Read the model definition and answer for the solid it produces. Units are mm, in the model's axes. Coordinates: 2 decimals unless noted, no trailing zeros. Write each loop counter-clockwise with the first axis right and the second up, starting at its lowest first coordinate (ties: lowest second). Pieces come first, ordered by that corner, then holes.
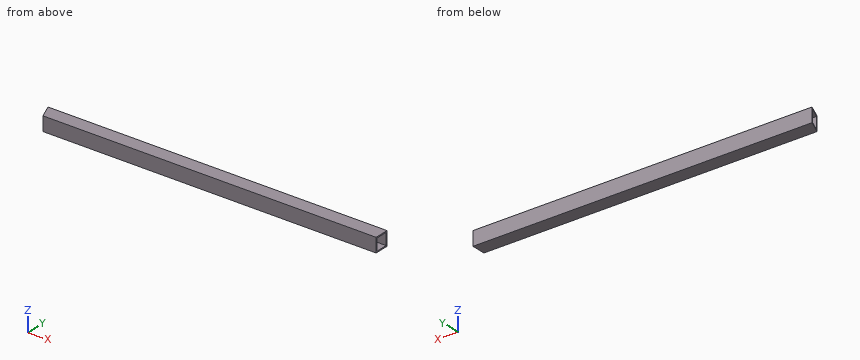
from build123d import *

# Parameters (mm, degrees)
F0_W        = 25
F0_H        = 25
F0_W_2      = 21
F0_H_2      = 21
F1_DEPTH    = 600
F2_T1_DEPTH = 180.5602235744


# Not quite as in the source:
# - a fillet or chamfer that OpenCascade refuses, or shapes differently, is made with other operations: its cross-section is extruded or revolved along the edge and cut away or added


with BuildPart() as f1:
    # F0 (on Right) → F1 (new body)
    with BuildSketch(Plane.YZ):
        Rectangle(F0_W, F0_H)
        Rectangle(F0_W_2, F0_H_2, mode=Mode.SUBTRACT)
    extrude(amount=F1_DEPTH)

    # F2: chamfer of 30 x 12.4264068712 on 1 edges, made by hand

    # F2_s2 → F2_t1 (cut)
    with BuildSketch(Plane.XY.offset(-90.2801117872)):
        Polygon((12.4264068712, -12.5), (0, 17.5), (0, -12.5), align=None)
    extrude(amount=F2_T1_DEPTH, mode=Mode.SUBTRACT)


solid = f1.part
Item 1: The part is cut by section C-C (y = -3). Give the vertices of the cut face in (x, z), and give its area (3 significant figures).
Item 2: Find the intervals of material crossed by probe 1 along Z at (x, y) = (469, 8.5); probe 2 along X at (y, z) = (-7, 10.75), in increasing order.
Item 3: The part is cut by section A-A (z = -3.75). Give the vertices of the cut face in (x, y), and give its area (3 significant figures).
Item 4: The part is cut by section B-B (x = 404.5). Give the vertices of the cut face in (y, z), and give its area (3 significant figures).
Answer:
1. outline: (8.49, -12.5) - (600, -12.5) - (600, -10.5) - (8.49, -10.5) - close; (8.49, 10.5) - (600, 10.5) - (600, 12.5) - (8.49, 12.5) - close
1. area: 2,370 mm2
2. probe 1: z = -12.5 to -10.5, 10.5 to 12.5
2. probe 2: x = 10.15 to 600
3. outline: (2.07, 12.5) - (2.9, 10.5) - (600, 10.5) - (600, 12.5) - close; (11.6, -10.5) - (12.43, -12.5) - (600, -12.5) - (600, -10.5) - close
3. area: 2,370 mm2
4. outline: (-12.5, -12.5) - (12.5, -12.5) - (12.5, 12.5) - (-12.5, 12.5) - close; hole (-10.5, -10.5) - (10.5, -10.5) - (10.5, 10.5) - (-10.5, 10.5) - close
4. area: 184 mm2
